from build123d import *

# Parameters (mm, degrees)
BOSS_EXTRUDE1_DEPTH = 4.3
CUT_EXTRUDE1_START  = 0.8
SKETCH2_OUTSIDE_W   = 17.962
SKETCH2_OUTSIDE_H   = 9.922
CUT_EXTRUDE1_DEPTH  = 4.5
FILLET1_R           = 0.4
CUT_EXTRUDE2_START  = 0.6
SKETCH3_OUTSIDE_W   = 17.962
SKETCH3_OUTSIDE_H   = 9.922
CUT_EXTRUDE2_DEPTH  = 4.7
SKETCH5_W           = 15.203925075
SKETCH5_H           = 7.601962538
CUT_EXTRUDE3_DEPTH  = 0.1
SKETCH6_W           = 4.55
SKETCH6_H           = 0.8
BOSS_EXTRUDE2_DEPTH = 0.3


with BuildPart() as part:
    # Sketch1 → Boss-Extrude1 (new body)
    with BuildSketch(Plane.XY):
        with BuildLine():
            Line((-4.019954666, 2.5), (4.019954666, 2.5))
            ThreePointArc((4.019954666, 2.5), (6.519954666, 0), (4.019954666, -2.5))
            Line((4.019954666, -2.5), (-4.019954666, -2.5))
            ThreePointArc((-4.019954666, -2.5), (-6.519954666, 0), (-4.019954666, 2.5))
        make_face()
    extrude(amount=BOSS_EXTRUDE1_DEPTH)

    # Sketch2 outside → Cut-Extrude1 (cut, through all)
    with BuildSketch(Plane.XY.offset(CUT_EXTRUDE1_START)):
        Rectangle(SKETCH2_OUTSIDE_W, SKETCH2_OUTSIDE_H)
        with BuildLine():
            Line((-4.019954666, 1.9), (4.019954666, 1.9))
            ThreePointArc((4.019954666, 1.9), (5.919954666, 0), (4.019954666, -1.9))
            Line((4.019954666, -1.9), (-4.019954666, -1.9))
            ThreePointArc((-4.019954666, -1.9), (-5.919954666, 0), (-4.019954666, 1.9))
        make_face(mode=Mode.SUBTRACT)
    extrude(amount=CUT_EXTRUDE1_DEPTH, mode=Mode.SUBTRACT)

    # Fillet1
    fillet1_edges = [part.edges().sort_by_distance(p)[0] for p in [
        (-5.919954666, 0, 4.3),
        (0, -1.9, 4.3),
        (5.919954666, 0, 4.3),
        (0, 1.9, 4.3),
    ]]
    fillet(fillet1_edges, radius=FILLET1_R)

    # Sketch3 outside → Cut-Extrude2 (cut, through all)
    with BuildSketch(Plane.XY.offset(CUT_EXTRUDE2_START)):
        Rectangle(SKETCH3_OUTSIDE_W, SKETCH3_OUTSIDE_H)
        with BuildLine():
            Line((-4.019954666, 2.3), (4.019954666, 2.3))
            ThreePointArc((4.019954666, 2.3), (6.319954666, 0), (4.019954666, -2.3))
            Line((4.019954666, -2.3), (-4.019954666, -2.3))
            ThreePointArc((-4.019954666, -2.3), (-6.319954666, 0), (-4.019954666, 2.3))
        make_face(mode=Mode.SUBTRACT)
    extrude(amount=CUT_EXTRUDE2_DEPTH, mode=Mode.SUBTRACT)

    # Sketch5 → Cut-Extrude3 (cut)
    with BuildSketch(Plane.XY):
        with Locations((0.247324124, -0.273358242)):
            Rectangle(SKETCH5_W, SKETCH5_H)
    extrude(amount=CUT_EXTRUDE3_DEPTH, mode=Mode.SUBTRACT)

    # Sketch6 → Boss-Extrude2 (add)
    with BuildSketch(Plane.XY):
        with Locations((-4.475, 0)):
            Rectangle(SKETCH6_W, SKETCH6_H)
        with Locations((4.475, 0)):
            Rectangle(SKETCH6_W, SKETCH6_H)
    extrude(amount=BOSS_EXTRUDE2_DEPTH)


solid = part.part
Verification items for the finished model (mm, model axes). A direction names the side the tool comes from. Coordinates: 2 decimals unless noted, no trailing zeros. Loops run counter-clockwise (first coordinate to the right, second up) from the corner with the lowest first, then second, coordinate; pieces in that order, holes last. Notation, with made-up numbers: (11, -32.75) -> (22, -32.75) arc R30 ccw to (22, 1.25) -> close; hole circle Ø5 at (50.5, 38). An arc over 180 degrees is marked (long way). Answer as CSV lines item,"result".
1) Thickness scan on L1, parallel to Z at x = -1.5, y = -0.9; L2, parallel to Y at x = 3.5, z = 2.7; L3, parallel to Z at x = 6.25, y = -0.3. Record the ranges inside material, lowest first. Write a range as from..to.
Found:
L1,"z = 0.1..4.3"
L2,"y = -1.9..1.9"
L3,"z = 0..0.8"
2) Tool access check on faces 1 (the flat face through (-0.5, 2.1, 0.8)), 2 (the cylindrical face through (-5.92, -0.04, 2.33)), 3 (the flat face through (0, -1.9, 2)), 4 (the flat face through (0, 1.9, 2)). Record the directions out of +Z, -Z, +X, -X, +Y, -Y that give a thin tool (end or side, any length) a straight path to the whole face; none if there is none.
Found:
face 1,"+Z"
face 2,"+Z, -X"
face 3,"+Z, +X, -X, -Y"
face 4,"+Z, +X, -X, +Y"
3) Depth check by flat-ended pin: pin 1 (0.9 mm diameter, centred on x = -2, z = 2.5, fed in from +Y). Enter the tip coordinate at first touch or a pass-through.
Found:
pin 1,"stops at y = 1.9"
4) Cross-section at B-B, the plane z = 1.5. Record the cut outline in (x, y).
Found:
outline,"(-4.02, -1.9) -> (4.02, -1.9) arc R1.9 ccw to (4.02, 1.9) -> (-4.02, 1.9) arc R1.9 ccw to start"
5) Cross-section at A-A, the plane y = 0. Record the cut outline in (x, z).
Found:
outline,"(-6.75, 0) -> (-2.2, 0) -> (-2.2, 0.1) -> (2.2, 0.1) -> (2.2, 0) -> (6.75, 0) -> (6.75, 0.3) -> (6.52, 0.3) -> (6.52, 0.6) -> (6.32, 0.6) -> (6.32, 0.8) -> (5.92, 0.8) -> (5.92, 3.9) arc R0.4 ccw to (5.52, 4.3) -> (-5.52, 4.3) arc R0.4 ccw to (-5.92, 3.9) -> (-5.92, 0.8) -> (-6.32, 0.8) -> (-6.32, 0.6) -> (-6.52, 0.6) -> (-6.52, 0.3) -> (-6.75, 0.3) -> close"
